Design review of the part shown in the three views and the two pictorial views. Dimensions are in mm from the part's minimum x, y and z. A direction names the side the tool comes from. Coordinates: 2 decimals unless noted, no trailing zeros. Loops run counter-clockwise (first coordinate to the right, second up) from the corner with the lowest first, then second, coordinate; pieces in that order, holes last. Notation, with made-up numbers: (89.25, -27.5) -> (140.25, -27.5) arc R18 cw to (140.25, -13.5) -> close; hole circle Ø2 at (-31, 68.5). An arc over 180 degrees is marked (long way). Answer in a Markdown table with one row per item.
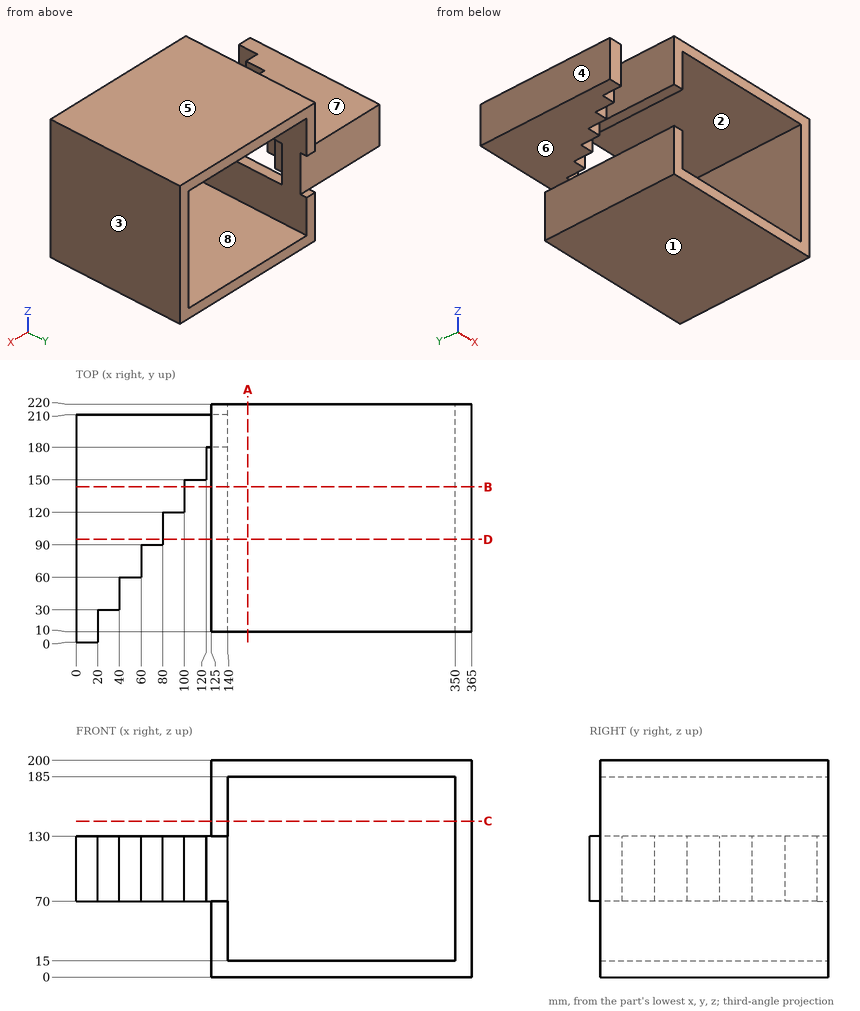
Item 1: The part is to be moulded in two halves that separate along Z. For the marked faces 1, 2 and 3, say which applies: +Z half, -Z half, draft (parallel to the pull), parting line (faces both ways), or undercut.
Worked answers:
| item | result |
|---|---|
| face 1 | -Z half |
| face 2 | undercut |
| face 3 | draft |
Item 2: For L1, parallel to X at y = 156, z = 90.5; L2, parallel to Z at x = 196.5, y = 208; L3, parallel to X at y = 140.5, z = 94.5, list the stretches that pass through material, from the lowest coordinate up.
Worked answers:
| item | result |
|---|---|
| L1 | 0 to 120, 350 to 365 |
| L2 | 0 to 15, 185 to 200 |
| L3 | 0 to 100, 350 to 365 |
Item 3: Insertion check: pin 1 (10 mm diameter, centred on x = 129, z = 108.5, fed in from -Y); pin 2 (16 mm diameter, centred on x = 73.5, z = 113.5, fed in from -Y); pin 3 (16 mm diameter, centred on x = 91, z = 114, fed in from -Y). Each pin has a flat end and moves straight along its axis. Give the tip position at first contact, or say it passes through.
Worked answers:
| item | result |
|---|---|
| pin 1 | y = 180 |
| pin 2 | y = 90 |
| pin 3 | y = 120 |
Item 4: Take a section at B-B, the plane y = 143.5. State the section outline as (x, z) points.
Worked answers:
| item | result |
|---|---|
| outline | (0, 70) -> (100, 70) -> (100, 130) -> (0, 130) -> close; (125, 0) -> (365, 0) -> (365, 200) -> (125, 200) -> (125, 130) -> (140, 130) -> (140, 185) -> (350, 185) -> (350, 15) -> (140, 15) -> (140, 70) -> (125, 70) -> close |
Item 5: For the marked faces 4, 5, 6, 7 and 8, list the 3-axis set-ups (+Z, -Z, +X, -X, +Y, -Y) from which the entire face can be reached by the end or side of a thin tool; tool diameter is ignored.
Worked answers:
| item | result |
|---|---|
| face 4 | +Z, -Z, -X, +Y, -Y |
| face 5 | +Z, +X, -X, +Y, -Y |
| face 6 | -Z, -X, +Y, -Y |
| face 7 | +Z, -X, +Y, -Y |
| face 8 | +Y, -Y |
Item 6: Take a section at A-A, the plane x = 158.5. State the section outline as (y, z) points, and give its area (3 significant figures).
Worked answers:
| item | result |
|---|---|
| outline | (10, 0) -> (220, 0) -> (220, 15) -> (10, 15) -> close; (10, 185) -> (220, 185) -> (220, 200) -> (10, 200) -> close |
| area | 6,300 mm² |
Item 7: Take a section at C-C, the plane z = 144. State the section outline as (x, y) points, and give its area (3 significant figures).
Worked answers:
| item | result |
|---|---|
| outline | (125, 10) -> (140, 10) -> (140, 220) -> (125, 220) -> close; (350, 10) -> (365, 10) -> (365, 220) -> (350, 220) -> close |
| area | 6,300 mm² |
Item 8: Take a section at D-D, the plane y = 95. State the section outline as (x, z) points.
Worked answers:
| item | result |
|---|---|
| outline | (0, 70) -> (80, 70) -> (80, 130) -> (0, 130) -> close; (125, 0) -> (365, 0) -> (365, 200) -> (125, 200) -> (125, 130) -> (140, 130) -> (140, 185) -> (350, 185) -> (350, 15) -> (140, 15) -> (140, 70) -> (125, 70) -> close |
